Check sheet for the modelled part. Datum: model origin and axes. Units: mm. A direction names the side the tool comes from. Give positions to 0.01 mm unless a question says otherwise; leave off trailing zeros. Order: outer loops, then holes, each group sorted by start corner. A loop starts at its lowest first (then second) coordinate and runs counter-clockwise, first axis right, second up.
from build123d import *

# Parameters (mm, degrees)
BOSS_EXTRUDE2_DEPTH     = 10
BOSS_EXTRUDE3_DEPTH     = 40
CUT_EXTRUDE3_DEPTH      = 51.268999561
CUT_EXTRUDE3_DEPTH_BACK = 40
CUT_EXTRUDE4_DEPTH      = 10


with BuildPart() as part:
    # Sketch1 → Boss-Extrude2 (new body)
    with BuildSketch(Plane.XY):
        with BuildLine():
            Line((-2.416609195, 3.25), (2.416609195, 3.25))
            ThreePointArc((2.416609195, 3.25), (4.05, 0), (2.416609195, -3.25))
            Line((2.416609195, -3.25), (-2.416609195, -3.25))
            ThreePointArc((-2.416609195, -3.25), (-4.05, 0), (-2.416609195, 3.25))
        make_face()
    extrude(amount=BOSS_EXTRUDE2_DEPTH)

    # Sketch4 → Boss-Extrude3 (add)
    with BuildSketch(Plane.XY.offset(10)):
        Polygon((1.87443765, -3.251125471), (3.752776074, -0.002252112), (1.878338424, 3.248873359), (-1.87443765, 3.251125471), (-3.752776074, 0.002252112), (-1.878338424, -3.248873359), align=None)
    extrude(amount=BOSS_EXTRUDE3_DEPTH)

    # Sketch5 → Cut-Extrude3 (cut, two sides: drawn at the far end of the back side and taken through both)
    with BuildSketch(Plane.XY.offset(50).offset(-CUT_EXTRUDE3_DEPTH_BACK)):
        Polygon((-1.300388139, -2.249220017), (1.297687604, -2.250779172), (2.598075744, -0.001559155), (1.300388139, 2.249220017), (-1.297687604, 2.250779172), (-2.598075744, 0.001559155), align=None)
    extrude(amount=CUT_EXTRUDE3_DEPTH + CUT_EXTRUDE3_DEPTH_BACK, mode=Mode.SUBTRACT)

    # Sketch3 → Cut-Extrude4 (cut)
    with BuildSketch(Plane(origin=(0, 0, 0), x_dir=(-1, 0, 0), z_dir=(0, 0, -1))):
        with BuildLine():
            Line((1.854723699, 1.75), (-1.854723699, 1.75))
            ThreePointArc((-1.854723699, 1.75), (-2.55, 0), (-1.854723699, -1.75))
            Line((-1.854723699, -1.75), (1.854723699, -1.75))
            ThreePointArc((1.854723699, -1.75), (2.55, 0), (1.854723699, 1.75))
        make_face()
    extrude(amount=-CUT_EXTRUDE4_DEPTH, mode=Mode.SUBTRACT)


solid = part.part
1) Set-up check for faces 4 (the face through (4.05, 0.05, 4.93)), 5 (the face through (2.55, 0.03, 4.93)), 6 (the face through (3.7, 0.5, 10)), 7 (the face through (2.8, -1.65, 29.72)), 8 (the face through (-1.958, -1.108, 29.72)): record each of +Z, -Z, +X, -X, +Y, -Y from which the full face is reachable in a straight line by a thin tool's end or side.
Recorded:
face 4: +Z, -Z, +X
face 5: -Z
face 6: +Z, +X
face 7: +Z, +X, -Y
face 8: +Z
2) Depth check by flat-ended pin: pin 1 Ø0.6 at (x, y) = (0.5, 2) entering from +Z. Enter the tip coordinate at first touch or a pass-through.
Recorded:
pin 1: stops at z = 50
3) Section check C-C, the plane y = -1. Record the cut outline in (x, z).
Recorded:
outline: (-3.92, 0) - (-2.35, 0) - (-2.35, 10) - (-2.02, 10) - (-2.02, 50) - (-3.17, 50) - (-3.17, 10) - (-3.92, 10) - close; (2.02, 10) - (2.35, 10) - (2.35, 0) - (3.92, 0) - (3.92, 10) - (3.18, 10) - (3.18, 50) - (2.02, 50) - close
4) Material ranges on L1, parallel to Y at x = -1, z = 30.5; L2, parallel to X at y = 1, z = 11.5, recorded low to high.
Recorded:
L1: y = -3.25 to -2.25, 2.25 to 3.25
L2: x = -3.18 to -2.02, 2.02 to 3.17
5) Section check A-A, the plane z = 14. Record the cut outline in (x, y).
Recorded:
outline: (-3.75, 0) - (-1.88, -3.25) - (1.87, -3.25) - (3.75, 0) - (1.88, 3.25) - (-1.87, 3.25) - close; hole (-2.6, 0) - (-1.3, -2.25) - (1.3, -2.25) - (2.6, 0) - (1.3, 2.25) - (-1.3, 2.25) - close
6) Draft check along X on faces 1 (the face through (2.2, 1, 50)), 2 (the face through (-2.83, -1.6, 29.72)), 3 (the face through (-2.55, -0.03, 4.93)). Enter one of: +X half, -X half, draft (parallel to the pull), parting line (faces both ways), or undercut.
Recorded:
face 1: draft
face 2: -X half
face 3: undercut
